```python
from build123d import *

# Parameters (mm, degrees)
F1_DEPTH = 25.4
F2_R     = 5.08


with BuildPart() as f1:
    # F0 (on Front) → F1 (new body)
    with BuildSketch(Plane.XZ):
        with BuildLine():
            Line((0, 43.18), (0, 0))
            Line((0, 0), (5.08, 0))
            Line((5.08, 0), (5.08, 34.925))
            ThreePointArc((5.08, 34.925), (6.009936, 37.170064), (8.255, 38.1))
            Line((8.255, 38.1), (55.245, 38.1))
            ThreePointArc((55.245, 38.1), (57.490064, 37.170064), (58.42, 34.925))
            Line((58.42, 34.925), (58.42, -63.5))
            Line((58.42, -63.5), (90.17, -63.5))
            Line((90.17, -63.5), (90.17, -38.1))
            Line((90.17, -38.1), (85.09, -38.1))
            Line((85.09, -38.1), (85.09, -52.07))
            ThreePointArc((85.09, -52.07), (83.230128, -56.560128), (78.74, -58.42))
            Line((78.74, -58.42), (69.85, -58.42))
            ThreePointArc((69.85, -58.42), (65.359872, -56.560128), (63.5, -52.07))
            Line((63.5, -52.07), (63.5, 43.18))
            Line((63.5, 43.18), (0, 43.18))
        make_face()
    extrude(amount=F1_DEPTH)

    # F2
    f2_edges = [f1.edges().sort_by_distance(p)[0] for p in [
        (0, -12.7, 43.18),
        (63.5, -12.7, 43.18),
        (90.17, -12.7, -63.5),
        (58.42, -12.7, -63.5),
    ]]
    fillet(f2_edges, radius=F2_R)


solid = f1.part
```
Verification items for the finished model (mm, model axes). A direction names the side the tool comes from. Round coordinates to 2 decimals unless told otherwise and drop trailing zeros. Write each loop counter-clockwise with the first axis right and the second up, starting at its lowest first coordinate (ties: lowest second). Pieces come first, ordered by that corner, then holes. Notation, with made-up numbers: (39.5, -8) - (87.5, -8) arc R20 ccw to (87.5, 16) - close; hole circle Ø4 at (-39.5, 71.5). An arc over 180 degrees is marked (long way). Answer as a JSON object with one key per item and string values. Group by question number.
Q1. Section check C-C, the plane z = -36. Enter the section's corners in (x, y).
Q2. Mould release check, pull along X, two halves, no side actions. Record for faces 1 (the flat face through (5.08, -13, 17)), 2 (the flat face through (3, -13, 0)), 3 (the cylindrical face through (88.642, -12.878, -62.051)): released by +X, released by -X, zero draft, split by the parting line, or undercut.
Q3. Section check B-B, the plane y = -18.25. Enter the section's corners in (x, z) (3 decimals), plus the area to 3 significant figures.
Q4. Section check D-D, the plane x = 48.5. Enter the section's corners in (y, z), plus the area to 3 significant figures.
Q5. Thickness scan on line 1 (X direction, y = -9.75, z = 23.5); line 2 (X direction, y = -23, z = -48.5); line 3 (Z direction, x = 31, y = -4). Record the ranges inside material, lowest first.
Q6. Tool access check on faces 4 (the cylindrical face through (83.28, -12.52, -56.51)), 5 (the flat face through (32, -13, 43.18)), 6 (the flat face through (62, 0, 2)), 7 (the cylindrical face through (57.47, -12.52, 37.19)), 8 (the flat face through (88, -13, -38.1)). Record the directions out of +Z, -Z, +X, -X, +Y, -Y that give a thin tool (end or side, any length) a straight path to the whole face; none if there is none.
Q7. Go/stop test with flat-tipped pins: pin 1 Ø7 at (y, z) = (-8, -47.5) entering from -X; pin 2 Ø5.5 at (x, y) = (2, -7) entering from -Z; pin 3 Ø4.5 at (x, y) = (72.5, -8.5) entering from +Z. Record where each tip stops, or that it passes through.
Q8. Section check A-A, the plane z = -54. Enter the section's corners in (x, y).
Found:
{
 "1": {"outline": "(58.42, -25.4) - (63.5, -25.4) - (63.5, 0) - (58.42, 0) - close"},
 "2": {"face 1": "undercut", "face 2": "zero draft", "face 3": "released by +X"},
 "3": {"outline": "(0, 0) - (5.08, 0) - (5.08, 34.925) arc R3.175 cw to (8.255, 38.1) - (55.245, 38.1) arc R3.175 cw to (58.42, 34.925) - (58.42, -58.42) arc R5.08 ccw to (63.5, -63.5) - (85.09, -63.5) arc R5.08 ccw to (90.17, -58.42) - (90.17, -38.1) - (85.09, -38.1) - (85.09, -52.07) arc R6.35 cw to (78.74, -58.42) - (69.85, -58.42) arc R6.35 cw to (63.5, -52.07) - (63.5, 38.1) arc R5.08 ccw to (58.42, 43.18) - (5.08, 43.18) arc R5.08 ccw to (0, 38.1) - close", "area": "1,270 mm^2"},
 "4": {"outline": "(-25.4, 38.1) - (0, 38.1) - (0, 43.18) - (-25.4, 43.18) - close", "area": "129 mm^2"},
 "5": {"line 1": "x = 0 to 5.08, 58.42 to 63.5", "line 2": "x = 58.42 to 63.5, 85.09 to 90.17", "line 3": "z = 38.1 to 43.18"},
 "6": {"face 4": "+Z, +Y, -Y", "face 5": "+Z, +X, -X, +Y, -Y", "face 6": "+Z, -Z, +X, -X, +Y", "face 7": "-Z, +Y, -Y", "face 8": "+Z, +X, +Y, -Y"},
 "7": {"pin 1": "stops at x = 58.42", "pin 2": "stops at z = 0", "pin 3": "stops at z = -58.42"},
 "8": {"outline": "(58.42, -25.4) - (63.8, -25.4) - (63.8, 0) - (58.42, 0) - close; (84.79, -25.4) - (90.17, -25.4) - (90.17, 0) - (84.79, 0) - close"}
}
